The model under review builds one solid part; all positions refer to its coordinate system, in mm. A direction names the side the tool comes from. Round coordinates to 2 decimals unless told otherwise and drop trailing zeros. Loops run counter-clockwise (first coordinate to the right, second up) from the corner with the lowest first, then second, coordinate; pieces in that order, holes last. Notation, with made-up numbers: M 17.5,-18.5 L 64.5,-18.5 A19 ccw 64.5,-2.5 Z; hole C -4.5,45.25 d7. An arc over 180 degrees is marked long. Use a Markdown table: item, result. Add a question column.
```python
from build123d import *

# Parameters (mm, degrees)
BOSS_EXTRUDE1_DEPTH             = 5.2
SKETCH2_R                       = 29
CUT_EXTRUDE1_DEPTH              = 5.2
SKETCH5_W                       = 6
SKETCH5_H                       = 15
BOSS_EXTRUDE3_DEPTH             = 15
SKETCH8_R                       = 5
CUT_EXTRUDE3_DEPTH              = 2
SKETCH9_R                       = 4
CUT_EXTRUDE4_DEPTH              = 191.628670456
BOSS_EXTRUDE2_DEPTH             = 24.8
CUT_EXTRUDE2_DEPTH              = 183.5
SKETCH15_W                      = 68
SKETCH15_H                      = 30
CUT_EXTRUDE5_DEPTH              = 10
SKETCH16_W                      = 6
SKETCH16_H                      = 45
BOSS_EXTRUDE4_DEPTH             = 40
CUT_EXTRUDE6_DEPTH              = 40
SKETCH19_W                      = 12
SKETCH19_H                      = 40
CUT_EXTRUDE7_DEPTH              = 40
F_4_0MM_DOWEL_HOLE2_D           = 4.2
SKETCH24_W                      = 110
SKETCH24_H                      = 2.5
BOSS_EXTRUDE5_DEPTH             = 40
SKETCH25_W                      = 68
SKETCH25_H                      = 5.2
BOSS_EXTRUDE6_DEPTH             = 3
SKETCH26_W                      = 18
SKETCH26_H                      = 15
SKETCH26_W_2                    = 6
BOSS_EXTRUDE7_DEPTH             = 15
SKETCH27_R                      = 4
CUT_EXTRUDE8_DEPTH              = 58
SKETCH28_R                      = 5
CUT_EXTRUDE9_DEPTH              = 2
LPATTERN1_COUNT                 = 2
LPATTERN1_PITCH                 = 18
LPATTERN2_COUNT                 = 2
LPATTERN2_PITCH                 = 92
LPATTERN2_COPY_1_SKETCH_R       = 5
LPATTERN2_COPY_1_DEPTH          = 2
F_4_0MM_DOWEL_HOLE1_D           = 4
F_4_0MM_DOWEL_HOLE1_DEPTH       = 8
F_4_0MM_DOWEL_HOLE1_CSINK_D     = 4.05
F_4_0MM_DOWEL_HOLE1_CSINK_ANGLE = 90
F_4_0MM_DOWEL_HOLE1_TIP         = 1.201721238


with BuildPart() as part:
    # Sketch1 → Boss-Extrude1 (new body)
    with BuildSketch(Plane(origin=(0, 0, 0), x_dir=(1, 0, 0), z_dir=(0, 1, 0))):
        Polygon((-70, -142.5), (70, -142.5), (70, -117.5), (70, 92.5), (55, 92.5), (55, 107.5), (-55, 107.5), (-55, 92.5), (-70, 92.5), (-70, -127.5), align=None)
    extrude(amount=BOSS_EXTRUDE1_DEPTH)

    # Sketch2 → Cut-Extrude1 (cut)
    with BuildSketch(Plane(origin=(0, 5.2, 0), x_dir=(1, 0, 0), z_dir=(0, 1, 0))):
        with Locations(Location((0, -32.5, 0), (0, 0, 270))):
            Circle(SKETCH2_R)
    extrude(amount=-CUT_EXTRUDE1_DEPTH, mode=Mode.SUBTRACT)

    # Sketch5 → Boss-Extrude3 (add)
    with BuildSketch(Plane(origin=(0, 5.2, 0), x_dir=(1, 0, 0), z_dir=(0, 1, 0))):
        with Locations((52, 100)):
            Rectangle(SKETCH5_W, SKETCH5_H)
        with Locations((-52, 100)):
            Rectangle(SKETCH5_W, SKETCH5_H)
    extrude(amount=BOSS_EXTRUDE3_DEPTH)

    # Sketch8 → Cut-Extrude3 (cut, symmetric)
    with BuildSketch(Plane.ZY.offset(52)):
        with Locations((-100, 20.2)):
            Circle(SKETCH8_R)
    cut_extrude3 = extrude(amount=CUT_EXTRUDE3_DEPTH, both=True, mode=Mode.SUBTRACT)

    # Mirror1: Cut-Extrude3 across plane
    add(cut_extrude3.mirror(Plane.ZY), mode=Mode.SUBTRACT)

    # Sketch9 → Cut-Extrude4 (cut, through all)
    with BuildSketch(Plane.ZY.offset(55)):
        with Locations((-100, 20.2)):
            Circle(SKETCH9_R)
    extrude(amount=-CUT_EXTRUDE4_DEPTH, mode=Mode.SUBTRACT)

    # Sketch3 → Boss-Extrude2 (add)
    with BuildSketch(Plane(origin=(0, 5.2, 0), x_dir=(1, 0, 0), z_dir=(0, 1, 0))):
        Polygon((-34, -32.5), (-34, -111.5), (-40, -111.5), (-40, 68.5), (-34, 68.5), align=None)
        Polygon((40, 68.5), (34, 68.5), (34, -32.5), (34, -111.5), (40, -111.5), align=None)
    extrude(amount=BOSS_EXTRUDE2_DEPTH)

    # Sketch4 → Cut-Extrude2 (cut, through all)
    with BuildSketch(Plane(origin=(40, 0, 0), x_dir=(0, 0, -1), z_dir=(1, 0, 0))):
        with BuildLine():
            Line((-111.5, 21.5), (38.5, 21.5))
            ThreePointArc((38.5, 21.5), (39.8, 20.2), (38.5, 18.9))
            Line((38.5, 18.9), (-111.5, 18.9))
            ThreePointArc((-111.5, 18.9), (-112.8, 20.2), (-111.5, 21.5))
        make_face()
    extrude(amount=-CUT_EXTRUDE2_DEPTH, mode=Mode.SUBTRACT)

    # Cut-Sweep4: sweep along a curve in space
    with BuildLine() as cut_sweep4_path:
        Line((40, 18.9, 111.5), (40, 18.9, -38.5))
    # Sketch10 → Cut-Sweep4 (sweep, cut)
    with BuildSketch(Plane.XY.offset(111.5)):
        with BuildLine():
            Line((36.5, 18.5), (36.5, 18.9))
            Line((36.5, 18.9), (37.5, 18.9))
            Line((37.5, 18.9), (37.5, 18.5))
            ThreePointArc((37.5, 18.5), (37, 18), (36.5, 18.5))
        make_face()
    cut_sweep4 = sweep(path=cut_sweep4_path.line, mode=Mode.SUBTRACT)

    # Mirror2: Cut-Sweep4 across plane
    add(cut_sweep4.mirror(Plane.ZY), mode=Mode.SUBTRACT)

    # Sketch15 → Cut-Extrude5 (cut)
    with BuildSketch(Plane(origin=(0, 5.2, 0), x_dir=(1, 0, 0), z_dir=(0, 1, 0))):
        with Locations((0, 30)):
            Rectangle(SKETCH15_W, SKETCH15_H)
    extrude(amount=-CUT_EXTRUDE5_DEPTH, mode=Mode.SUBTRACT)

    # Sketch16 → Boss-Extrude4 (add)
    with BuildSketch(Plane.XZ):
        with Locations((31, -70)):
            Rectangle(SKETCH16_W, SKETCH16_H)
    extrude(amount=BOSS_EXTRUDE4_DEPTH)

    # Sketch17 → Cut-Extrude6 (cut)
    with BuildSketch(Plane.ZY.offset(-28)):
        with BuildLine():
            Line((-85.4, -5), (-85.4, -35))
            ThreePointArc((-85.4, -35), (-87.5, -37.1), (-89.6, -35))
            Line((-89.6, -35), (-89.6, -5))
            ThreePointArc((-89.6, -5), (-87.5, -2.9), (-85.4, -5))
        make_face()
        with BuildLine():
            Line((-50.4, -5), (-50.4, -35))
            ThreePointArc((-50.4, -35), (-52.5, -37.1), (-54.6, -35))
            Line((-54.6, -35), (-54.6, -5))
            ThreePointArc((-54.6, -5), (-52.5, -2.9), (-50.4, -5))
        make_face()
        with BuildLine():
            Line((-63, -10), (-63, -30))
            ThreePointArc((-63, -30), (-70, -37), (-77, -30))
            Line((-77, -30), (-77, -10))
            ThreePointArc((-77, -10), (-70, -3), (-63, -10))
        make_face()
    extrude(amount=-CUT_EXTRUDE6_DEPTH, mode=Mode.SUBTRACT)

    # Sketch19 → Cut-Extrude7 (cut)
    with BuildSketch(Plane.XZ):
        with Locations((22, -82.5)):
            Rectangle(SKETCH19_W, SKETCH19_H)
    extrude(amount=-CUT_EXTRUDE7_DEPTH, mode=Mode.SUBTRACT)

    # Ø4.0mm Dowel Hole2 (through all)
    with Locations(Plane(origin=(0, 5.2, 0), x_dir=(1, 0, 0), z_dir=(0, 1, 0))):
        with Locations((-62.5, 82.5), (62.5, 82.5), (62.5, -87.5), (-62.5, -87.5)):
            Hole(F_4_0MM_DOWEL_HOLE2_D / 2)

    # Sketch24 → Boss-Extrude5 (add)
    with BuildSketch(Plane.XZ):
        with Locations((0, -46.25)):
            Rectangle(SKETCH24_W, SKETCH24_H)
    extrude(amount=BOSS_EXTRUDE5_DEPTH)

    # Sketch25 → Boss-Extrude6 (add)
    with BuildSketch(Plane.XY.offset(-45)):
        with Locations((0, 2.6)):
            Rectangle(SKETCH25_W, SKETCH25_H)
    extrude(amount=BOSS_EXTRUDE6_DEPTH)

    # Sketch26 → Boss-Extrude7 (add)
    with BuildSketch(Plane(origin=(0, 5.2, 0), x_dir=(1, 0, 0), z_dir=(0, 1, 0))):
        with Locations((-61, -135)):
            Rectangle(SKETCH26_W, SKETCH26_H)
        with Locations((61, -135)):
            Rectangle(SKETCH26_W, SKETCH26_H)
        with Locations((-37, -135)):
            Rectangle(SKETCH26_W_2, SKETCH26_H)
        with Locations((37, -135)):
            Rectangle(SKETCH26_W_2, SKETCH26_H)
    extrude(amount=BOSS_EXTRUDE7_DEPTH)

    # Sketch27 → Cut-Extrude8 (cut, symmetric)
    with BuildSketch(Plane.ZY):
        with Locations((135, 20.2)):
            Circle(SKETCH27_R)
    extrude(amount=CUT_EXTRUDE8_DEPTH, both=True, mode=Mode.SUBTRACT)

    # Sketch28 → Cut-Extrude9 (cut, symmetric)
    with BuildSketch(Plane(origin=(-55, 0, 0), x_dir=(0, 0, -1), z_dir=(1, 0, 0))):
        with Locations((-135, 20.2)):
            Circle(SKETCH28_R)
    cut_extrude9 = extrude(amount=CUT_EXTRUDE9_DEPTH, both=True, mode=Mode.SUBTRACT)

    # LPattern1: Cut-Extrude9 ×2
    with Locations(*[(i * LPATTERN1_PITCH, 0, 0) for i in range(1, LPATTERN1_COUNT)]):
        add(cut_extrude9, mode=Mode.SUBTRACT)

    # LPattern2: Cut-Extrude9 ×2
    with Locations(*[(i * LPATTERN2_PITCH, 0, 0) for i in range(1, LPATTERN2_COUNT)]):
        add(cut_extrude9, mode=Mode.SUBTRACT)

    # LPattern2 copy 1 sketch → LPattern2 copy 1 (cut, symmetric)
    with BuildSketch(Plane(origin=(55, 0, 0), x_dir=(0, 0, -1), z_dir=(1, 0, 0))):
        with Locations((-135, 20.2)):
            Circle(LPATTERN2_COPY_1_SKETCH_R)
    extrude(amount=LPATTERN2_COPY_1_DEPTH, both=True, mode=Mode.SUBTRACT)

    # Ø4.0mm Dowel Hole1
    with Locations(Plane(origin=(0, 20.2, 0), x_dir=(1, 0, 0), z_dir=(0, 1, 0))):
        with Locations((-63, -134.5), (63, -134.5)):
            CounterSinkHole(F_4_0MM_DOWEL_HOLE1_D / 2, F_4_0MM_DOWEL_HOLE1_CSINK_D / 2, depth=F_4_0MM_DOWEL_HOLE1_DEPTH, counter_sink_angle=F_4_0MM_DOWEL_HOLE1_CSINK_ANGLE)
            with Locations((0, 0, -(F_4_0MM_DOWEL_HOLE1_DEPTH + F_4_0MM_DOWEL_HOLE1_TIP / 2))):  # 118° drill point
                Cone(0, F_4_0MM_DOWEL_HOLE1_D / 2, F_4_0MM_DOWEL_HOLE1_TIP, mode=Mode.SUBTRACT)


solid = part.part
```
(1) To check wall thickness, follow probe 1 along Z at (x, y) = (-62.5, 2.25); probe 2 along X at (y, z) = (3.4, 87.5); probe 3 along X at (y, z) = (14.75, 134.5). State the ranges of each line that lie inside material, in increasing order.
(2) Consider section A-A, the plane z = -100. Give the boundary of the cut face in (x, y).
(3) Insertion check: pin 1 Ø1.5 at (y, z) = (17, -97.5) entering from -X; pin 2 Ø1.8 at (x, z) = (-52, -93.5) entering from +Y; pin 3 Ø5.5 at (y, z) = (18.5, -99) entering from +X. Each pin has a flat end and moves straight along its axis. Give the tip position at first contact, or say it passes through.
(4) For faces 4 (the face through (34, 13, 135)), 5 (the face through (-1, -20, -45)), 6 (the face through (-39, 16, 135)), 7 (the face through (31, -20, -77)), list the 3-axis set-ups (+Z, -Z, +X, -X, +Y, -Y) from which the entire face can be reached by the end or side of a thin tool; tool diameter is ignored.
(5) Consider section B-B, the plane y = 2.5. Give the boundary of the cut face in (x, z).
(6) Consider section C-C, the plane x = 0. Give the boundary of the cut face in (y, z).
(7) Draft analysis for pull direction X (two halves, no side actions). For faces 1 (the face through (-40, 17, 23)), 2 (the face through (-1, 3, 142.5)), 3 (the face through (30, 5.2, 16)), state which applies: released by +X, released by -X, zero draft, split by the parting line, or undercut.
Found:
| question | item | result |
|---|---|---|
| 1 | probe 1 | z = -92.5 to -84.6, -80.4 to 85.4, 89.6 to 142.5 |
| 1 | probe 2 | x = -70 to -64.6, -60.4 to 60.4, 64.6 to 70 |
| 1 | probe 3 | x = -70 to -65, -61 to -52, -40 to -34, 34 to 40, 52 to 61, 65 to 70 |
| 2 | outline | M -55,0 L 16,0 L 16,5.2 L -49,5.2 L -49,16.2 L -50,16.2 L -50,15.2 L -54,15.2 L -54,16.2 L -55,16.2 Z; M 28,0 L 55,0 L 55,16.2 L 54,16.2 L 54,15.2 L 50,15.2 L 50,16.2 L 49,16.2 L 49,5.2 L 28,5.2 Z |
| 3 | pin 1 | stops at x = -55 |
| 3 | pin 2 | stops at y = 20.2 |
| 3 | pin 3 | stops at x = 55 |
| 4 | face 4 | +Z, -Z, +Y |
| 4 | face 5 | +Z, +X, -X, -Y |
| 4 | face 6 | +Y |
| 4 | face 7 | +X, -X |
| 5 | outline | M -70,-92.5 L -55,-92.5 L -55,-107.5 L 55,-107.5 L 55,-92.5 L 70,-92.5 L 70,142.5 L -70,142.5 Z; hole C -62.5,-82.5 d4.2; hole C -62.5,87.5 d4.2; hole M -34,-42 L 34,-42 L 34,-15 L -34,-15 Z; hole C 0,32.5 d58; hole M 16,-102.5 L 28,-102.5 L 28,-62.5 L 16,-62.5 Z; hole C 62.5,-82.5 d4.2; hole C 62.5,87.5 d4.2 |
| 6 | outline | M -40,-47.5 L 0,-47.5 L 0,-107.5 L 5.2,-107.5 L 5.2,-42 L 0,-42 L 0,-45 L -40,-45 Z; M 0,-15 L 5.2,-15 L 5.2,3.5 L 0,3.5 Z; M 0,61.5 L 5.2,61.5 L 5.2,142.5 L 0,142.5 Z |
| 7 | face 1 | released by -X |
| 7 | face 2 | zero draft |
| 7 | face 3 | undercut |
